Build history of the part. All positions in model axes, mm. A direction names the side the tool comes from. Coordinates: 2 decimals unless noted, no trailing zeros. Order: outer loops, then holes, each group sorted by start corner. A loop starts at its lowest first (then second) coordinate and runs counter-clockwise, first axis right, second up. Notation, with made-up numbers: M 25,56 L 40,56 A10 ccw 40,67 Z; hole C -8,32 d6. An arc over 180 degrees is marked long. Use a Markdown table: item, result. Add a question column.
from build123d import *

# Parameters (mm, degrees)
SKETCH_W      = 100
SKETCH_H      = 100
PAD_DEPTH     = 2
SKETCH002_W   = 100
SKETCH002_H   = 100
SKETCH002_W_2 = 88.711022
SKETCH002_H_2 = 87.098678
PAD001_DEPTH  = 40
SKETCH003_W   = 27.317078
SKETCH003_H   = 6.504059
POCKET_DEPTH  = 7


with BuildPart() as part:
    # Sketch → Pad (new body)
    with BuildSketch(Plane.XY):
        Rectangle(SKETCH_W, SKETCH_H)
    extrude(amount=PAD_DEPTH)

    # Sketch002 (on Face6 of Pad) → Pad001 (join)
    with BuildSketch(Plane.XY.offset(2)):
        Rectangle(SKETCH002_W, SKETCH002_H)
        Rectangle(SKETCH002_W_2, SKETCH002_H_2, mode=Mode.SUBTRACT)
    extrude(amount=PAD001_DEPTH)

    # Sketch003 (on Face8 of Pad001) → Pocket (cut)
    with BuildSketch(Plane.XZ.offset(50)):
        with Locations((-16.619589, 28.616544)):
            Rectangle(SKETCH003_W, SKETCH003_H)
    extrude(amount=-POCKET_DEPTH, mode=Mode.SUBTRACT)


solid = part.part
(1) Slice it at D-D on z = 30.5. Give the cut face in (x, y).
(2) Which spindle directions (+Z, -Z, +X, -X, +Y, -Y) get a long thin tool onto all of the face, cutting with end or side? Do faces 1 (the flat face through (50, -1, 21)), 2 (the flat face through (44.356, -1, 22)), 3 (the flat face through (-30.278, -47, 29)). Say none if no direction does.
(3) Drill centre lines: line 1 along X through (y, z) = (38, 23); line 2 along Y through (x, z) = (-27.5, 16); line 3 along Z through (x, y) = (-9, 43). Where is each one in solid material? Low to high. Write a range as from..to.
(4) Mould opens along Z. For faces 4 (the flat face through (-1, 1, 0)), 5 (the flat face through (-1, 43.549, 22)), 6 (the flat face through (-17, -47, 31.869)) say: released by +Z, released by -Z, zero draft, split by the parting line, or undercut.
(5) Slice it at B-B on z = 22. Give the cut face in (x, y).
(6) Slice it at A-A on x = -5.5. Give the cut face in (y, z).
(7) Drop flat-ended pins along their axis: P1, Ø1.9, axis at x = -19, y = -47.5, coming from the -Z side; P2, Ø8, axis at x = 8, y = -23.5, coming from the +Z side. Give the stop position or say it passes through.
(8) Slice it at C-C on y = 7. Give the cut face in (x, z), and give its area (3 significant figures).
Solutions:
| question | item | result |
|---|---|---|
| 1 | outline | M -50,-50 L -30.28,-50 L -30.28,-43.55 L -44.36,-43.55 L -44.36,43.55 L 44.36,43.55 L 44.36,-43.55 L -2.96,-43.55 L -2.96,-50 L 50,-50 L 50,50 L -50,50 Z |
| 2 | face 1 | +Z, -Z, +X, +Y, -Y |
| 2 | face 2 | +Z |
| 2 | face 3 | -Y |
| 3 | line 1 | -50..-44.36, 44.36..50 |
| 3 | line 2 | -50..-43.55, 43.55..50 |
| 3 | line 3 | 0..2 |
| 4 | face 4 | released by -Z |
| 4 | face 5 | zero draft |
| 4 | face 6 | undercut |
| 5 | outline | M -50,-50 L 50,-50 L 50,50 L -50,50 Z; hole M -44.36,-43.55 L 44.36,-43.55 L 44.36,43.55 L -44.36,43.55 Z |
| 6 | outline | M -50,0 L 50,0 L 50,42 L 43.55,42 L 43.55,2 L -43.55,2 L -43.55,25.36 L -50,25.36 Z; M -50,31.87 L -43.55,31.87 L -43.55,42 L -50,42 Z |
| 7 | P1 | z = 0 |
| 7 | P2 | z = 2 |
| 8 | outline | M -50,0 L 50,0 L 50,42 L 44.36,42 L 44.36,2 L -44.36,2 L -44.36,42 L -50,42 Z |
| 8 | area | 652 mm² |
